from build123d import *

# Parameters (mm, degrees)
ESQUISSE1_W                  = 66
ESQUISSE1_H                  = 57.75
BOSS_EXTRU_1_DEPTH           = 0.8
CONG_1_R                     = 5.5
ESQUISSE3_W                  = 4
ESQUISSE3_H                  = 27.25
ESQUISSE3_W_2                = 6.5
ESQUISSE3_H_2                = 4.5
ESQUISSE3_W_3                = 2
ESQUISSE3_H_3                = 4
ENL_V_MAT_EXTRU_1_DEPTH      = 1.8
ENL_V_MAT_EXTRU_1_DEPTH_BACK = 1.8
CONG_2_R                     = 0.25
CONG_3_R                     = 0.5


with BuildPart() as part:
    # Esquisse1 → Boss.-Extru.1 (new body, symmetric)
    with BuildSketch(Plane(origin=(0, 0, 0), x_dir=(1, 0, 0), z_dir=(0, 1, 0))):
        Rectangle(ESQUISSE1_W, ESQUISSE1_H)
    extrude(amount=BOSS_EXTRU_1_DEPTH, both=True)

    # Congé1
    cong_1_edges = [part.edges().sort_by_distance(p)[0] for p in [
        (33, 0, 28.875),
        (-33, 0, 28.875),
        (-33, 0, -28.875),
        (33, 0, -28.875),
    ]]
    fillet(cong_1_edges, radius=CONG_1_R)

    # Esquisse3 → Enlèv. mat.-Extru.1 (cut, two sides)
    with BuildSketch(Plane(origin=(0, 0, 0), x_dir=(1, 0, 0), z_dir=(0, 1, 0))) as enl_v_mat_extru_1_sk:
        with Locations((-33, 1.245)):
            Rectangle(ESQUISSE3_W, ESQUISSE3_H)
        with Locations((33, -12.875)):
            Rectangle(ESQUISSE3_W_2, ESQUISSE3_H_2)
        with Locations((-11, 28.875)):
            Rectangle(ESQUISSE3_W_3, ESQUISSE3_H_3)
        with Locations((29, 28.875)):
            Rectangle(ESQUISSE3_W_3, ESQUISSE3_H_3)
        with Locations((30, -28.875)):
            Rectangle(ESQUISSE3_W_3, ESQUISSE3_H_3)
        with Locations((33, 12.875)):
            Rectangle(ESQUISSE3_W_2, ESQUISSE3_H_2)
    extrude(amount=ENL_V_MAT_EXTRU_1_DEPTH, mode=Mode.SUBTRACT)
    extrude(enl_v_mat_extru_1_sk.sketch, amount=-ENL_V_MAT_EXTRU_1_DEPTH_BACK, mode=Mode.SUBTRACT)

    # Congé2
    cong_2_edges = [part.edges().sort_by_distance(p)[0] for p in [
        (30, 0, -26.875),
        (28, 0, -26.875),
        (33, 0, 10.625),
        (29.75, 0, 10.625),
        (33, 0, 15.125),
        (29.75, 0, 15.125),
        (29, 0, 28.666502622),
        (28, 0, -28.852225575),
        (30, 0, -28.273979486),
        (-33, 0, 12.38),
        (-31, 0, 12.38),
        (-33, 0, -14.87),
        (-31, 0, -14.87),
        (33, 0, -10.625),
        (33, 0, -15.125),
        (29.75, 0, -15.125),
        (29.75, 0, -10.625),
        (-10, 0, -28.875),
        (-12, 0, -28.875),
        (-12, 0, -26.875),
        (-10, 0, -26.875),
        (31, 0, 26.875),
        (29, 0, 26.875),
    ]]
    fillet(cong_2_edges, radius=CONG_2_R)

    # Congé3
    cong_3_edges = [part.edges().sort_by_distance(p)[0] for p in [
        (31, 0, 27.617640687),
    ]]
    fillet(cong_3_edges, radius=CONG_3_R)


solid = part.part
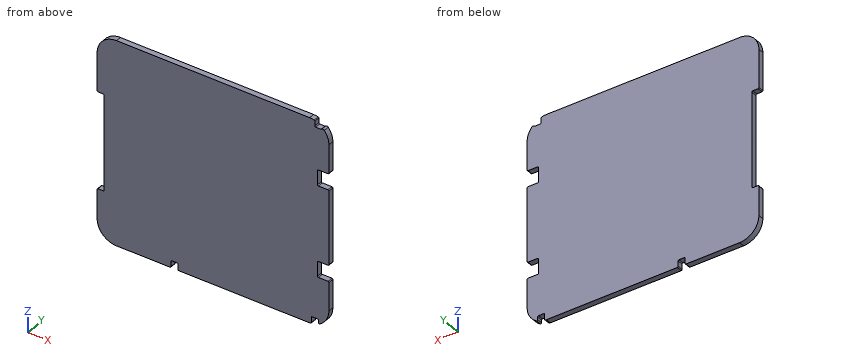
Input: part model. Units: mm. Frame: model coordinates. Coordinates: 2 decimals unless noted, no trailing zeros. Loops run counter-clockwise (first coordinate to the right, second up) from the corner with the lowest first, then second, coordinate; pieces in that order, holes last. Notation, with made-up numbers: (7.5, 60.25) - (30.5, 60.25) arc R16 ccw to (30.5, 91.25) - close; hole circle Ø7 at (1.5, 3.5). An arc over 180 degrees is marked (long way). Answer in a Markdown table with one row per item. Add a question column.
Item 1: Contact query for flat-ended pins moving along their axis: P1, Ø0.7, axis at y = 0.5, z = -28, coming from the +X side; P2, Ø0.5, axis at x = 31.5, y = 0, coming from the +Z side; P3, Ø0.8, axis at y = -0.5, z = 12, coming from the +X side. Output: stop coordinate, or through.
Item 2: Line query: line 1 along X through (y, z) = (-0.55, 14); line 2 along X through (y, z) = (-0.1, -11); line 3 along Z through (x, y) = (-28, -0.45). Output: solid intervals per line, ascending. Write a range as [from, to].
Item 3: Section query A-A on z = -6. Return the cut outline in (x, y), then the cut area to 3 significant figures.
Recorded:
| question | item | result |
|---|---|---|
| 1 | P1 | x = 30.96 |
| 1 | P2 | z = 27.12 |
| 1 | P3 | x = 29.75 |
| 2 | line 1 | [-33, 29.75] |
| 2 | line 2 | [-31, 29.75] |
| 2 | line 3 | [-28.85, 28.85] |
| 3 | outline | (-31, -0.8) - (33, -0.8) - (33, 0.8) - (-31, 0.8) - close |
| 3 | area | 102 mm^2 |
